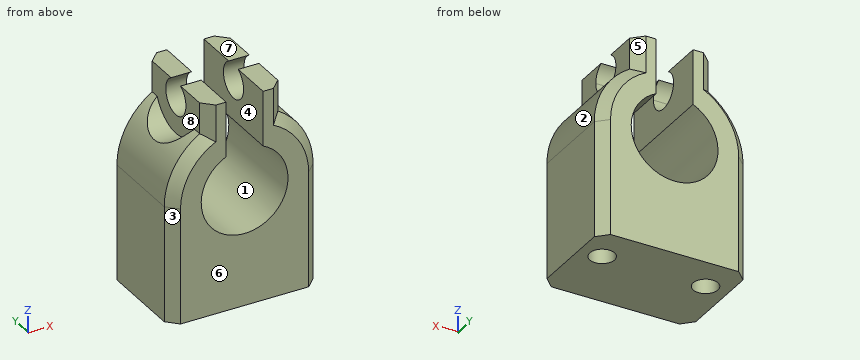
```python
from build123d import *

# Parameters (mm, degrees)
F1_DEPTH = 10
F3_DEPTH = 4
F4_DEPTH = 20
F5_R     = 1.2
F6_DEPTH = 6
F7_SIZE  = 1


with BuildPart() as f1:
    # F0 (on Front) → F1 (new body)
    with BuildSketch(Plane.XZ):
        with BuildLine():
            ThreePointArc((1.7895, 3.7996960076), (0, -4.2), (-1.7895, 3.7996960076))
            Line((-1.7895, 3.7996960076), (-1.7895, 6.9740726803))
            Line((-1.7895, 6.9740726803), (-1.7895, 9.1220658074))
            Line((-1.7895, 9.1220658074), (-3.7895, 9.1220658074))
            Line((-3.7895, 9.1220658074), (-3.7895, 6.1220658074))
            ThreePointArc((-3.7895, 6.1220658074), (-6.2898489648, 3.5039691779), (-7.2, 0))
            Line((-7.2, 0), (-7.2, -11.2))
            Line((-7.2, -11.2), (7.2, -11.2))
            Line((7.2, -11.2), (7.2, 0))
            ThreePointArc((7.2, 0), (6.2898489648, 3.5039691779), (3.7895, 6.1220658074))
            Line((3.7895, 6.1220658074), (3.7895, 9.1220658074))
            Line((3.7895, 9.1220658074), (1.7895, 9.1220658074))
            Line((1.7895, 9.1220658074), (1.7895, 6.9740726803))
            Line((1.7895, 6.9740726803), (1.7895, 3.7996960076))
        make_face()
    extrude(amount=F1_DEPTH)

    # F2 (on face) → F3 (cut)
    with BuildSketch(Plane(origin=(-3.7895, 0, 0), x_dir=(0, -1, 0), z_dir=(-1, 0, 0))):
        with BuildLine():
            ThreePointArc((5.8, 9.1220658074), (6.4577379737, 8.4967085916), (6.7, 7.6220658074))
            ThreePointArc((6.7, 7.6220658074), (6.4577379737, 6.7474230232), (5.8, 6.1220658074))
            Line((5.8, 6.1220658074), (8.1622776602, 6.1220658074))
            ThreePointArc((8.1622776602, 6.1220658074), (8.4145257219, 6.8532913966), (8.5, 7.6220658074))
            ThreePointArc((8.5, 7.6220658074), (8.4145257219, 8.3908402182), (8.1622776602, 9.1220658074))
            Line((8.1622776602, 9.1220658074), (5.8, 9.1220658074))
        make_face()
        with BuildLine():
            ThreePointArc((4.2, 9.1220658074), (5, 9.3220658074), (5.8, 9.1220658074))
            Line((5.8, 9.1220658074), (8.1622776602, 9.1220658074))
            ThreePointArc((8.1622776602, 9.1220658074), (5, 11.1220658074), (1.8377223398, 9.1220658074))
            Line((1.8377223398, 9.1220658074), (4.2, 9.1220658074))
        make_face()
        with BuildLine():
            Line((8.1622776602, 6.1220658074), (5.8, 6.1220658074))
            ThreePointArc((5.8, 6.1220658074), (5, 5.9220658074), (4.2, 6.1220658074))
            Line((4.2, 6.1220658074), (1.8377223398, 6.1220658074))
            ThreePointArc((1.8377223398, 6.1220658074), (5, 4.1220658074), (8.1622776602, 6.1220658074))
        make_face()
        with BuildLine():
            ThreePointArc((4.2, 6.1220658074), (3.3, 7.6220658074), (4.2, 9.1220658074))
            Line((4.2, 9.1220658074), (1.8377223398, 9.1220658074))
            ThreePointArc((1.8377223398, 9.1220658074), (1.5, 7.6220658074), (1.8377223398, 6.1220658074))
            Line((1.8377223398, 6.1220658074), (4.2, 6.1220658074))
        make_face()
    extrude(amount=F3_DEPTH, mode=Mode.SUBTRACT)

    # F2 (on face) → F4 (cut, symmetric)
    with BuildSketch(Plane(origin=(-3.7895, 0, 0), x_dir=(0, -1, 0), z_dir=(-1, 0, 0))):
        with BuildLine():
            Line((4.2, 9.1220658074), (5.8, 9.1220658074))
            ThreePointArc((5.8, 9.1220658074), (5, 9.3220658074), (4.2, 9.1220658074))
        make_face()
        with BuildLine():
            ThreePointArc((5.8, 6.1220658074), (6.4577379737, 6.7474230232), (6.7, 7.6220658074))
            ThreePointArc((6.7, 7.6220658074), (6.4577379737, 8.4967085916), (5.8, 9.1220658074))
            Line((5.8, 9.1220658074), (4.2, 9.1220658074))
            ThreePointArc((4.2, 9.1220658074), (3.3, 7.6220658074), (4.2, 6.1220658074))
            Line((4.2, 6.1220658074), (5.8, 6.1220658074))
        make_face()
        with BuildLine():
            ThreePointArc((4.2, 6.1220658074), (5, 5.9220658074), (5.8, 6.1220658074))
            Line((5.8, 6.1220658074), (4.2, 6.1220658074))
        make_face()
    extrude(amount=F4_DEPTH, both=True, mode=Mode.SUBTRACT)

    # F5 (on face) → F6 (cut)
    with BuildSketch(Plane(origin=(0, 0, -11.2), x_dir=(1, 0, 0), z_dir=(0, 0, -1))):
        with Locations((-5, 3.5)):
            Circle(F5_R)
        with Locations((5, 3.5)):
            Circle(F5_R)
    extrude(amount=-F6_DEPTH, mode=Mode.SUBTRACT)

    # F7
    f7_edges = [f1.edges().sort_by_distance(p)[0] for p in [
        (7.2, 0, -5.6),
        (7.2, -10, -5.6),
        (-7.2, -10, -5.6),
        (-7.2, 0, -5.6),
        (3.7895, -10, 7.622066),
        (3.7895, 0, 7.622066),
        (-3.7895, -10, 7.622066),
        (-3.7895, 0, 7.622066),
        (-6.289849, 0, 3.503969),
        (6.289849, 0, 3.503969),
        (-6.289849, -10, 3.503969),
        (6.289849, -10, 3.503969),
    ]]
    chamfer(f7_edges, length=F7_SIZE)


solid = f1.part
```
Here's how the part is built. I have some questions about the finished solid (model axes, mm). Face numbers are marked on the shaded views. A direction names the side the tool comes from. Coordinates: 2 decimals unless noted, no trailing zeros. Write each loop counter-clockwise with the first axis right and the second up, starting at its lowest first coordinate (ties: lowest second). Pieces come first, ordered by that corner, then holes. Notation, with made-up numbers: (-19.5, 74) -> (29.5, 74) arc R28 ccw to (29.5, 96) -> close; hole circle Ø9 at (68.5, 80.5). An arc over 180 degrees is marked (long way). Use a Markdown table: item, result. Add a question column.
(1) If we section it at B-B, the plane y = -5: Write out the boundary of the cut face in (x, z).
(2) We'd pull the mould along X, two halves only. Please class the marked faces 1, 2 and 3: +X half, -X half, draft (parallel to the pull), parting line (faces both ways), or undercut.
(3) I'm going to push flat-ended pins straight in: P1, Ø3.5, axis at y = -8, z = 7.5, coming from the +X side; P2, Ø1.2, axis at x = 5, y = -3.5, coming from the -Z side; P3, Ø0.9, axis at y = -2.5, z = 8, coming from the +X side. Where does each tip first touch, or does it pass through?
(4) For the marked faces 4, 5, 6, 7 and 8, which set-ups out of +Z, -Z, +X, -X, +Y, -Y let a thin tool reach every point of the face, with its end or its side?
(5) If we section it at D-D, the plane x = 0: Write out the boundary of the cut face in (y, z), and give its area (3 significant figures).
(6) If we section it at A-A, the plane z = -9: Write out the boundary of the cut face in (x, y).
(7) Please list where these lines run through material, in increasing order: line 1 (X direction, y = -3.5, z = -8.75); line 2 (Y direction, x = -5, z = -7.4); line 3 (Y direction, x = -2.5, z = 8.25).
(8) If we section it at C-C, the plane z = -0.75: Write out the boundary of the cut face in (x, y).
Outcome:
| question | item | result |
|---|---|---|
| 1 | outline | (-7.2, -11.2) -> (7.2, -11.2) -> (7.2, 0) arc R7.2 ccw to (4.1, 5.92) -> (1.79, 5.92) -> (1.79, 3.8) arc R4.2 cw (long way) to (-1.79, 3.8) -> (-1.79, 5.92) -> (-3.79, 5.92) -> (-3.79, 4.12) -> (-5.9, 4.12) arc R7.2 ccw to (-7.2, 0) -> close |
| 2 | face 1 | undercut |
| 2 | face 2 | +X half |
| 2 | face 3 | -X half |
| 3 | P1 | stops at x = 4.33 |
| 3 | P2 | stops at z = -5.2 |
| 3 | P3 | stops at x = 3.79 |
| 4 | face 4 | +Z, +Y, -Y |
| 4 | face 5 | +Z, +X, +Y |
| 4 | face 6 | +Z, -Z, +X, -X, -Y |
| 4 | face 7 | +Z, +X, -X, +Y, -Y |
| 4 | face 8 | +Z, -X |
| 5 | outline | (-10, -11.2) -> (0, -11.2) -> (0, -4.2) -> (-10, -4.2) -> close |
| 5 | area | 70.0 mm^2 |
| 6 | outline | (-7.2, -9) -> (-6.2, -10) -> (6.2, -10) -> (7.2, -9) -> (7.2, -1) -> (6.2, 0) -> (-6.2, 0) -> (-7.2, -1) -> close; hole circle Ø2.4 at (-5, -3.5); hole circle Ø2.4 at (5, -3.5) |
| 7 | line 1 | x = -7.2 to -6.2, -3.8 to 3.8, 6.2 to 7.2 |
| 7 | line 2 | y = -10 to -4.7, -2.3 to 0 |
| 7 | line 3 | y = -10 to -6.58, -3.42 to 0 |
| 8 | outline | (-7.2, -9) -> (-6.2, -10) -> (-4.13, -10) -> (-4.13, 0) -> (-6.2, 0) -> (-7.2, -1) -> close; (4.13, -10) -> (6.2, -10) -> (7.2, -9) -> (7.2, -1) -> (6.2, 0) -> (4.13, 0) -> close |
